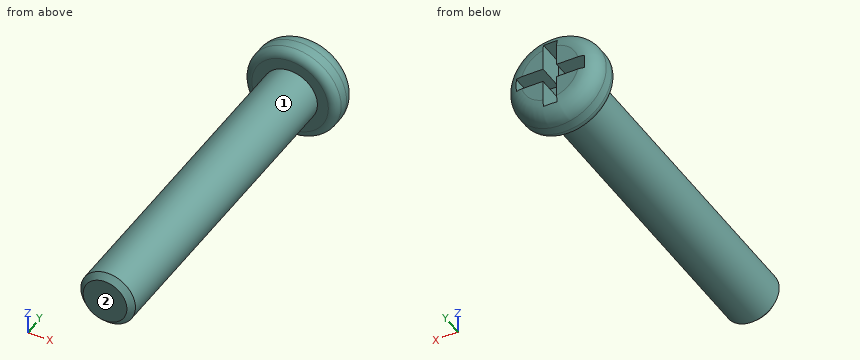
Autodesk Inventor part; units mm, degrees
ref_plane "YZ Plane" through (0, 0, 0) normal (1, 0, 0) x (0, 1, 0)
ref_plane "XZ Plane" through (0, 0, 0) normal (0, 1, 0) x (-1, 0, 0)
ref_plane "XY Plane" through (0, 0, 0) normal (0, 0, 1) x (1, 0, 0)
sketch "Sketch1" plane through (0, 0, 0) normal (0, 1, 0) x (-1, 0, 0)
  circle A0 centre (0, 0) radius 1
  dimension "d0" = 2
extrude "Extrusion1" add sketch "Sketch1" along normal blind 13.3
sketch "Sketch2" plane through (0, 13.3, 0) normal (0, 1, 0) x (1, 0, 0)
  circle A0 centre (0, 0) radius 1
  circle A1 centre (0, 0) radius 1.7
  dimension "d3" = 3.4
extrude "Extrusion2" add sketch "Sketch2" against normal blind 1.3 contours A0 | A1
thread "Thread1"
sketch "Sketch3" plane through (0, 13.3, 0) normal (0, 1, 0) x (1, 0, 0)
  line L0 (-1.25, -0.25) -> (1.25, -0.25)
  line L1 (1.25, -0.25) -> (1.25, 0.25)
  line L2 (1.25, 0.25) -> (-1.25, 0.25)
  line L3 (-1.25, 0.25) -> (-1.25, -0.25)
  line L4 (-1.25, -0.25) -> (1.25, 0.25) construction
  line L5 (1.25, -0.25) -> (-1.25, 0.25) construction
  line L6 (-0.25, 1.25) -> (0.25, 1.25)
  line L7 (0.25, 1.25) -> (0.25, -1.25)
  line L8 (0.25, -1.25) -> (-0.25, -1.25)
  line L9 (-0.25, -1.25) -> (-0.25, 1.25)
  circle A0 centre (0, 0) radius 1
  line L10 (-0.25, 1.25) -> (0.25, -1.25) construction
  line L11 (0.25, 1.25) -> (-0.25, -1.25) construction
  point P0 (-0.25, -0.25)
  point P1 (0.25, -0.25)
  point P2 (0.25, 0.25)
  point P3 (-0.25, 0.25)
  dimension "d8" = 2.5
  dimension "d9" = 0.5
  dimension "d10" = 0.5
  dimension "d11" = 2.5
extrude "Extrusion3" cut sketch "Sketch3" against normal blind 1 contours L3 L2 A0 L0 | A0 L2 L9 L0 | L9 L2 L7 L0 | L0 L7 A0 L9 | A0 L7 L8 L9 | L7 L2 A0 L0 | L9 A0 L7 L2 | L9 L6 L7 A0 | A0 L2 L1 L0
chamfer "Chamfer1" distance 0.2 angle 45 1 edges at (1, 0, 0)
fillet "Fillet1" radius 0.65 1 edges at (-1.7, 13.3, 0)
fillet "Fillet2" radius 0.3 1 edges at (-1.7, 12, 0)
properties part number "M2_Short_Bolt"
Input: part model. Units: mm. Frame: model coordinates. Face numbers are marked on the shaded views. A direction names the side the tool comes from. Coordinates: 2 decimals unless noted, no trailing zeros. Write each loop counter-clockwise with the first axis right and the second up, starting at its lowest first coordinate (ties: lowest second). Pieces come first, ordered by that corner, then holes. Notation, with made-up numbers: (60, -9) - (91, -9) arc R33 ccw to (91, 23) - close; hole circle Ø10 at (40.25, -27.5). An arc over 180 degrees is marked (long way). Put each result on its own line as item: value. Start each with the question number.
1) Contact query for flat-ended pins moving along their axis: pin 1 (0.5 mm diameter, centred on x = -0.5, y = 13, fed in from -Z); pin 2 (0.8 mm diameter, centred on x = -0.5, y = 12.5, fed in from +Z); pin 3 (0.5 mm diameter, centred on y = 13, z = -0.5, fed in from +X). Output: stop coordinate, or through.
2) Cut plane A-A (z = 0). Return the cut outline in (x, y).
3) Cut plane B-B (x = 0). Return the cut outline in (y, z).
4) Reachability of the marked faces 1 and 2 from +Z, -Z, +X, -X, +Y, -Y: full face, straight path, thin tool, end or side. Return the list, or none.
5) Ray query, L1, parallel to Y at x = 0, z = -0.6; L2, parallel to Y at x = 0.2, z = -1.1; L3, parallel to X at y = 9, z = 0.6. Return the intervals inside material, ascending.
6) Cut plane C-C (y = 10.75). Return the cut outline in (x, z).
Resolved:
1. pin 1: stops at z = -1.65
1. pin 2: stops at z = 1.7
1. pin 3: stops at x = 1.65
2. outline: (-1.7, 12.3) arc R0.3 ccw to (-1.4, 12) - (-1, 12) - (-1, 0.2) - (-0.8, 0) - (0.8, 0) - (1, 0.2) - (1, 12) - (1.4, 12) arc R0.3 ccw to (1.7, 12.3) - (1.7, 12.65) arc R0.65 ccw to (1.25, 13.27) - (1.25, 12.3) - (-1.25, 12.3) - (-1.25, 13.27) arc R0.65 ccw to (-1.7, 12.65) - close
3. outline: (0, -0.8) - (0.2, -1) - (12, -1) - (12, -1.4) arc R0.3 ccw to (12.3, -1.7) - (12.65, -1.7) arc R0.65 ccw to (13.27, -1.25) - (12.3, -1.25) - (12.3, 1.25) - (13.27, 1.25) arc R0.65 ccw to (12.65, 1.7) - (12.3, 1.7) arc R0.3 ccw to (12, 1.4) - (12, 1) - (0.2, 1) - (0, 0.8) - close
4. face 1: -Y
4. face 2: +Z, -Z, +X, -X, -Y
5. L1: y = 0 to 12.3
5. L2: y = 12 to 12.3
5. L3: x = -0.8 to 0.8
6. outline: circle Ø2 at (0, 0)
